Geometry: see drawing. Coordinates: mm, zero at the bounding-box minimum. Give positions to 0.01 mm unless a question says otherwise; leave off trailing zeros. Loops run counter-clockwise (first coordinate to the right, second up) from the corner with the lowest first, then second, coordinate; pieces in that order, holes last. Notation, with made-up numbers: (-6.5, 63) -> (5.5, 63) arc R5 cw to (5.5, 69) -> close; hole circle Ø7 at (39, 78). An arc over 180 degrees is marked (long way). Use CSV: the item, a comma, the result in double quotes.
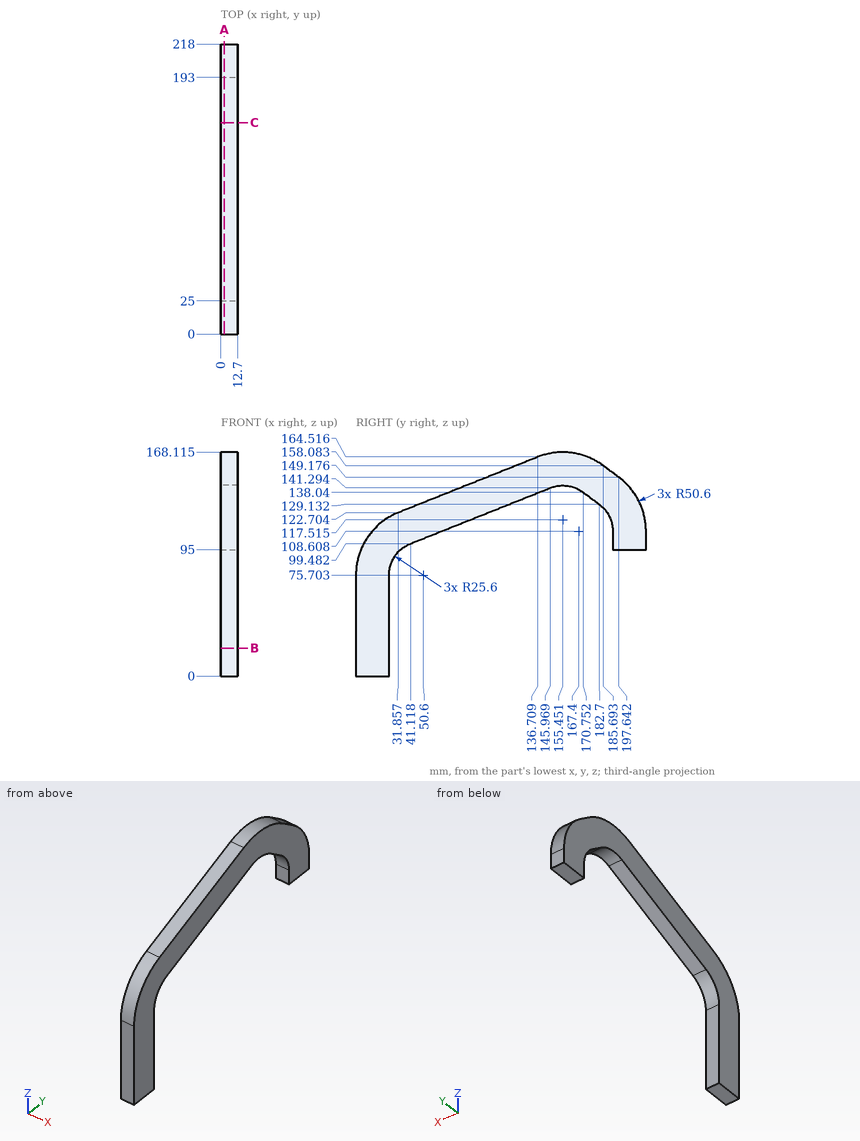
1) Ray query, line 1 (Y direction, x = 8, z = 56); line 2 (Z direction, x = 8.75, y = 112.5); line 3 (Z direction, x = 4.5, y = 102.5) (1 decimal). Return the intervals inside material, ascending.
From the geometry:
line 1,"y = 0 to 25"
line 2,"z = 127.95 to 154.86"
line 3,"z = 124 to 150.9"
2) Section query A-A (x = 2.5). Return loops of the section in (y, z) (1 decimal).
From the geometry:
outline,"(0, 0) -> (25, 0) -> (25, 75.7) arc R25.6 cw to (41.1, 99.5) -> (146, 141.3) arc R25.6 cw to (170.8, 138) -> (182.7, 129.1) arc R25.6 cw to (193, 108.6) -> (193, 95) -> (218, 95) -> (218, 108.6) arc R50.6 ccw to (197.6, 149.2) -> (185.7, 158.1) arc R50.6 ccw to (136.7, 164.5) -> (31.9, 122.7) arc R50.6 ccw to (0, 75.7) -> close"
3) Section query C-C (y = 159). Return loops of the section in (x, z).
From the geometry:
outline,"(0, 142.87) -> (12.7, 142.87) -> (12.7, 167.99) -> (0, 167.99) -> close"
4) Contact query for flat-ended pins moving along their axis: pin 1 (1.5 mm diameter, centred on x = 2.5, y = 35, fed in from +Z); pin 2 (3 mm diameter, centred on x = 4, y = 152, fed in from +Z); pin 3 (1.5 mm diameter, centred on x = 3, y = 140.5, fed in from -Z) (1 decimal). Output: stop coordinate, or through.
From the geometry:
pin 1,"stops at z = 124.26"
pin 2,"stops at z = 168.08"
pin 3,"stops at z = 138.8"
5) Section query B-B (z = 21). Return loops of the section in (x, y).
From the geometry:
outline,"(0, 0) -> (12.7, 0) -> (12.7, 25) -> (0, 25) -> close"
